Here's how the part is built. I have some questions about the finished solid (model axes, mm). Face numbers are marked on the shaded views. Coordinates: 2 decimals unless noted, no trailing zeros. Write each loop counter-clockwise with the first axis right and the second up, starting at its lowest first coordinate (ties: lowest second). Pieces come first, ordered by that corner, then holes. Notation, with made-up numbers: (-9, 83) -> (49, 83) arc R20 ccw to (49, 121) -> close; hole circle Ø2 at (52.5, -2). An arc over 180 degrees is marked (long way). Use a Markdown table: item, result. Add a question column.
Item 1: Will these pins go through, and if not, where does the flat tip stop? pin 1 Ø6 at (x, y) = (13, 21.5) entering from +Z; pin 2 Ø2 at (x, y) = (16.5, 16.5) entering from -Z; pin 3 Ø3 at (y, z) = (20, 67) entering from +X.
Item 2: Imagine slicing it at B-B, the plane z = 0. Write out the boundary of the cut face in (x, y), and give its area (3 significant figures).
Item 3: Imagine slicing it at C-C, the plane x = -10. Write out the boundary of the cut face in (y, z), and give its area (3 significant figures).
Item 4: Imagine slicing it at A-A, the plane y = 0. Write out the boundary of the cut face in (x, z).
Item 5: If we mould it in two halves opening along Z, with no side actions, what happens to the marked faces 1, 2 and 3? For each: pulls with the +Z half, pulls with the -Z half, needs draft (parallel to the pull), parting line crosses it, or undercut.
Item 6: Imagine slicing it at D-D, the plane z = 121.5. Write out the boundary of the cut face in (x, y).
Item 7: If I drill on line 1 along Z through (x, y) = (14, 0); line 2 along X through (y, z) = (11.5, 108.5), over which ranges is the centre line in solid material (lowest first)? Write a range as from..to.
```python
from build123d import *

# Parameters (mm, degrees)
SKETCH1_R           = 35
SKETCH1_R_2         = 25
BOSS_EXTRUDE1_DEPTH = 24
BOSS_EXTRUDE2_DEPTH = 7.5
SKETCH3_R           = 8
CUT_EXTRUDE1_DEPTH  = 15
CUT_EXTRUDE2_DEPTH  = 150.875815261
SKETCH6_R           = 4.5
CUT_EXTRUDE3_DEPTH  = 24


with BuildPart() as part:
    # Sketch1 → Boss-Extrude1 (new, symmetric)
    with BuildSketch(Plane(origin=(0, 0, 0), x_dir=(0, 0, -1), z_dir=(1, 0, 0))):
        Circle(SKETCH1_R)
        Circle(SKETCH1_R_2, mode=Mode.SUBTRACT)
    extrude(amount=BOSS_EXTRUDE1_DEPTH, both=True)

    # Sketch2 → Boss-Extrude2 (add, symmetric)
    with BuildSketch(Plane(origin=(0, 0, 0), x_dir=(0, 0, -1), z_dir=(1, 0, 0))):
        with BuildLine():
            Line((-18.027756377, 30), (-119.579019246, 19.901846216))
            ThreePointArc((-119.579019246, 19.901846216), (-137.6, 0), (-119.579019246, -19.901846216))
            Line((-119.579019246, -19.901846216), (-18.027756377, -30))
            ThreePointArc((-18.027756377, -30), (-35, 0), (-18.027756377, 30))
        make_face()
    extrude(amount=BOSS_EXTRUDE2_DEPTH, both=True)

    # Sketch3 → Cut-Extrude1 (cut)
    with BuildSketch(Plane(origin=(7.5, 0, 0), x_dir=(0, 0, -1), z_dir=(1, 0, 0))):
        with Locations((-117.6, 0)):
            Circle(SKETCH3_R)
    extrude(amount=-CUT_EXTRUDE1_DEPTH, mode=Mode.SUBTRACT)

    # Sketch5 → Cut-Extrude2 (cut, through all)
    with BuildSketch(Plane(origin=(24, 0, 0), x_dir=(0, 0, -1), z_dir=(1, 0, 0))):
        Polygon((-3.702856162, 6.196638775), (-25.314422766, -15.41492783), (-15.41492783, -25.314422766), (6.196638775, -3.702856162), align=None)
    extrude(amount=-CUT_EXTRUDE2_DEPTH, mode=Mode.SUBTRACT)

    # Sketch6 → Cut-Extrude3 (cut)
    with BuildSketch(Plane.XY.offset(-35)):
        with Locations(Location((0, 0, 0), (0, 0, 180))):
            Circle(SKETCH6_R)
    extrude(amount=CUT_EXTRUDE3_DEPTH, mode=Mode.SUBTRACT)


solid = part.part
```
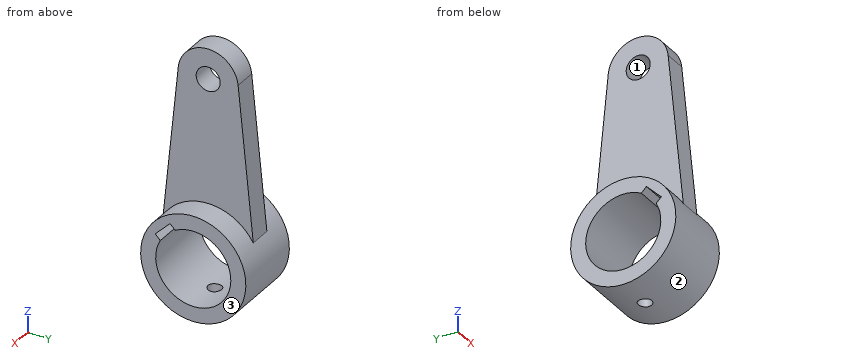
Ans:
| question | item | result |
|---|---|---|
| 1 | pin 1 | stops at z = 29.71 |
| 1 | pin 2 | stops at z = -31.38 |
| 1 | pin 3 | stops at x = 7.5 |
| 2 | outline | (-24, -35) -> (24, -35) -> (24, -25) -> (-24, -25) -> close; (-24, 25) -> (24, 25) -> (24, 35) -> (-24, 35) -> close |
| 2 | area | 960 mm^2 |
| 3 | outline | circle Ø70 at (0, 0); hole (-25.31, 15.41) -> (-21.92, 12.02) arc R25 ccw (long way) to (-12.02, 21.92) -> (-15.41, 25.31) -> close |
| 3 | area | 1,830 mm^2 |
| 4 | outline | (-24, -35) -> (-4.5, -35) -> (-4.5, -25) -> (-24, -25) -> close; (-24, 25) -> (24, 25) -> (24, 35) -> (7.5, 35) -> (7.5, 109.6) -> (-7.5, 109.6) -> (-7.5, 35) -> (-24, 35) -> close; (-7.5, 125.6) -> (7.5, 125.6) -> (7.5, 137.6) -> (-7.5, 137.6) -> close; (4.5, -35) -> (24, -35) -> (24, -25) -> (4.5, -25) -> close |
| 5 | face 1 | undercut |
| 5 | face 2 | parting line crosses it |
| 5 | face 3 | needs draft |
| 6 | outline | (-7.5, -19.62) -> (7.5, -19.62) -> (7.5, -6.98) -> (-7.5, -6.98) -> close; (-7.5, 6.98) -> (7.5, 6.98) -> (7.5, 19.62) -> (-7.5, 19.62) -> close |
| 7 | line 1 | z = -35..-25, 25..35 |
| 7 | line 2 | x = -7.5..7.5 |
